Build history of the part. All positions in model axes, mm. Face numbers are marked on the shaded views. Round coordinates to 2 decimals unless told otherwise and drop trailing zeros. Loops run counter-clockwise (first coordinate to the right, second up) from the corner with the lowest first, then second, coordinate; pieces in that order, holes last. Notation, with made-up numbers: (78, 41.25) - (119, 41.25) arc R20 cw to (119, 55.25) - close; hole circle Ø11 at (57, -25). An arc over 180 degrees is marked (long way). Put each result on its own line as item: value. Start each with the question number.
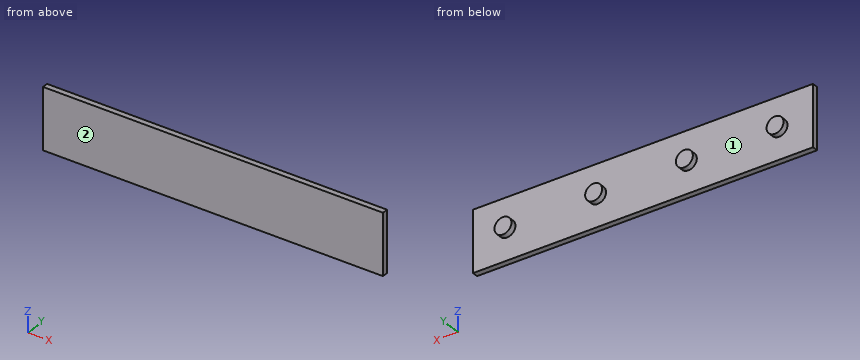
from build123d import *

# Parameters (mm, degrees)
SKETCH1_W           = 281.158896912
SKETCH1_H           = 50.8
BOSS_EXTRUDE1_DEPTH = 9.525
SKETCH2_OUTSIDE_W   = 340.332
SKETCH2_OUTSIDE_H   = 109.974
SKETCH2_OUTSIDE_R   = 7
CUT_EXTRUDE1_DEPTH  = 4.7625


with BuildPart() as part:
    # Sketch1 → Boss-Extrude1 (new body)
    with BuildSketch(Plane(origin=(0, 0, 0), x_dir=(1, 0, 0), z_dir=(0, 1, 0))):
        Rectangle(SKETCH1_W, SKETCH1_H)
    extrude(amount=BOSS_EXTRUDE1_DEPTH)

    # Sketch2 outside → Cut-Extrude1 (cut)
    with BuildSketch(Plane(origin=(0, 9.525, 0), x_dir=(1, 0, 0), z_dir=(0, 1, 0))):
        Rectangle(SKETCH2_OUTSIDE_W, SKETCH2_OUTSIDE_H)
        with Locations((-112.5, 0)):
            Circle(SKETCH2_OUTSIDE_R, mode=Mode.SUBTRACT)
        with Locations((-37.5, 0)):
            Circle(SKETCH2_OUTSIDE_R, mode=Mode.SUBTRACT)
        with Locations((37.5, 0)):
            Circle(SKETCH2_OUTSIDE_R, mode=Mode.SUBTRACT)
        with Locations((112.5, 0)):
            Circle(SKETCH2_OUTSIDE_R, mode=Mode.SUBTRACT)
    extrude(amount=-CUT_EXTRUDE1_DEPTH, mode=Mode.SUBTRACT)


solid = part.part
Item 1: Drop a flat-ended pin along its axis: pin 1 Ø8 at (x, z) = (15.5, 11.5) entering from +Y. Give the stop position or say it passes through.
Item 2: Two-plate mould, pull along X, no slides. Class the marked faces 1 and 2: pulls with the +X half, pulls with the -X half, needs draft (parallel to the pull), parting line crosses it, or undercut.
Item 3: Slice it at A-A (x = -113). Give the cut face in (y, z) (1 decimal), plus the area to 3 significant figures.
Item 4: Drill centre lines: probe 1 along X at (y, z) = (6, 5); probe 2 along Y at (x, z) = (86.5, -16); probe 3 along X at (y, z) = (8, -4). Where is each one in solid material? Low to high. Write a range as [from, to].
Item 5: Slice it at B-B (z = -3). Give the cut face in (x, y) (1 decimal), plus the area to 3 significant figures.
Item 6: Slice it at D-D (z = 22.5). Give the cut face in (x, y).
Computed values:
1. pin 1: stops at y = 4.76
2. face 1: undercut
2. face 2: needs draft
3. outline: (0, -25.4) - (4.8, -25.4) - (4.8, -7) - (9.5, -7) - (9.5, 7) - (4.8, 7) - (4.8, 25.4) - (0, 25.4) - close
3. area: 308 mm^2
4. probe 1: x = [-117.4, -107.6], [-42.4, -32.6], [32.6, 42.4], [107.6, 117.4]
4. probe 2: y = [0, 4.76]
4. probe 3: x = [-118.24, -106.76], [-43.24, -31.76], [31.76, 43.24], [106.76, 118.24]
5. outline: (-140.6, 0) - (140.6, 0) - (140.6, 4.8) - (118.8, 4.8) - (118.8, 9.5) - (106.2, 9.5) - (106.2, 4.8) - (43.8, 4.8) - (43.8, 9.5) - (31.2, 9.5) - (31.2, 4.8) - (-31.2, 4.8) - (-31.2, 9.5) - (-43.8, 9.5) - (-43.8, 4.8) - (-106.2, 4.8) - (-106.2, 9.5) - (-118.8, 9.5) - (-118.8, 4.8) - (-140.6, 4.8) - close
5. area: 1,580 mm^2
6. outline: (-140.58, 0) - (140.58, 0) - (140.58, 4.76) - (-140.58, 4.76) - close
